The drawing under review shows one solid part. Ordinate dimensions are in mm from its lowest x, y, z. Give positions to 0.01 mm unless a question says otherwise; leave off trailing zeros. Loops run counter-clockwise (first coordinate to the right, second up) from the corner with the lowest first, then second, coordinate; pieces in that order, holes last. Notation, with made-up numbers: (4.5, 6.25) - (37.5, 6.25) arc R4 cw to (37.5, 12.25) - close; hole circle Ø9 at (-25, 88). An arc over 180 degrees is marked (long way). Answer as CSV lines item,"result".
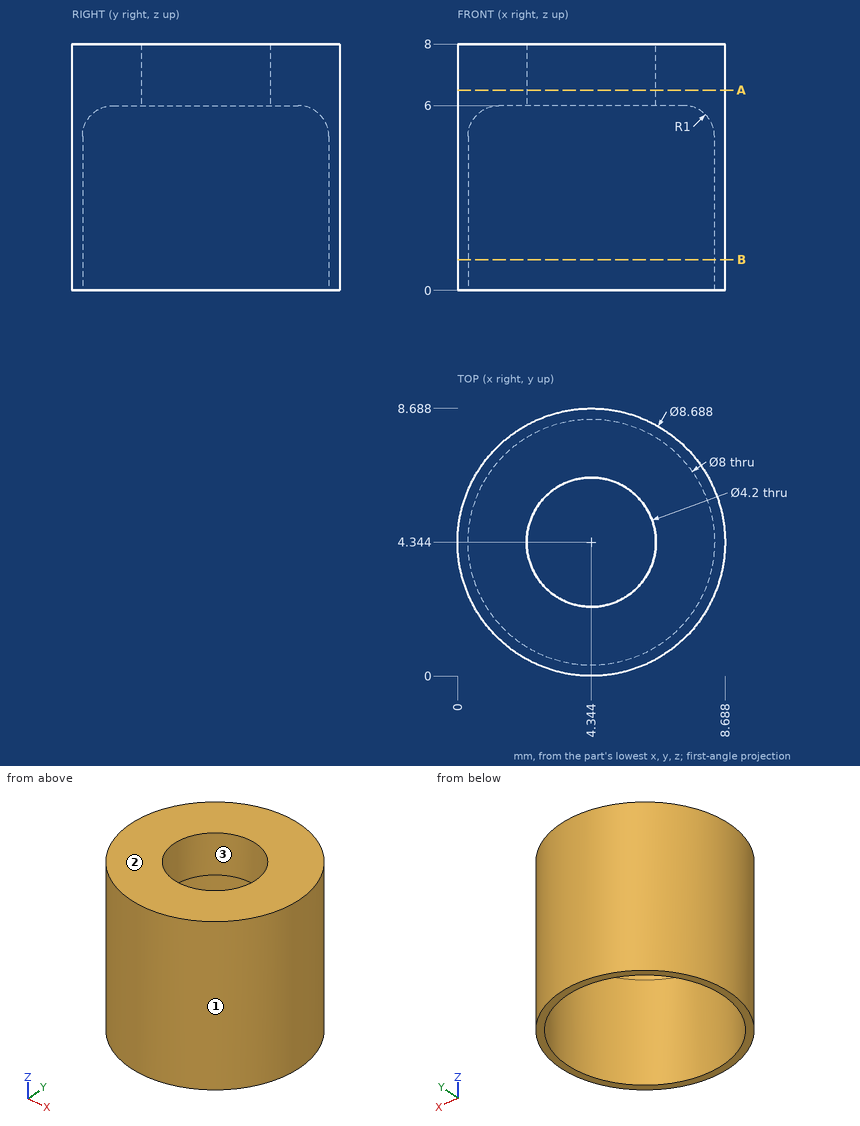
1) Draft analysis for pull direction X (two halves, no side actions). For the marked faces 1, 2 and 3, state which applies: pulls with the +X half, pulls with the -X half, needs draft (parallel to the pull), parting line crosses it, or undercut.
From the geometry:
face 1,"parting line crosses it"
face 2,"needs draft"
face 3,"undercut"
2) Consider section A-A on z = 6.5. Write out the cut boundary in (x, y).
From the geometry:
outline,"circle Ø8.69 at (4.34, 4.34); hole circle Ø4.2 at (4.34, 4.34)"
3) Consider section B-B on z = 1. Write out the cut boundary in (x, y).
From the geometry:
outline,"circle Ø8.69 at (4.34, 4.34); hole circle Ø8 at (4.34, 4.34)"
4) Insertion check: P1, Ø1.5, axis at y = 7, z = 1, coming from the +X side; P2, Ø1, axis at x = 6.5, y = 2, coming from the -Z side; P3, Ø4, axis at x = 7, z = 5.5, coming from the +Y side. Each pin has a flat end and moves straight along its axis. Give the tip position at first contact, or say it passes through.
From the geometry:
P1,"stops at x = 8.25"
P2,"stops at z = 5.73"
P3,"stops at y = 8.64"
5) Wall thickness on line 1 (X direction, y = 4.25, z = 5) (1 decimal); line 2 (Y direction, x = 5, z = 2); line 3 (X direction, y = 7.5, z = 4.25) (1 decimal): over which ranges is each line inside the solid? List them lowest first. Write a range as from..to.
From the geometry:
line 1,"x = 0..0.3, 8.3..8.7"
line 2,"y = 0.05..0.4, 8.29..8.64"
line 3,"x = 1.4..1.9, 6.8..7.3"
